Source: CAD feature listing. Evaluate the final solid. Frame: model axes, mm. A direction names the side the tool comes from. Round coordinates to 2 decimals unless told otherwise and drop trailing zeros. Order: outer loops, then holes, each group sorted by start corner. A loop starts at its lowest first (then second) coordinate and runs counter-clockwise, first axis right, second up. Notation, with made-up numbers: M 73,36 L 102,36 A22 ccw 102,42 Z; hole C -31,11.5 d9. An arc over 180 degrees is marked long. Answer in a Markdown table with one row per item. Add a question column.
```python
from build123d import *

# Parameters (mm, degrees)
SKETCH1_R          = 0.75
BASE_FLANGE1_DEPTH = 1


# Sheet-metal steps are written as plain solids
with BuildPart() as part:
    # Sketch1 → Base-Flange1 (new body)
    with BuildSketch(Plane.XY):
        with BuildLine():
            Line((-3.140050919, -11.322657825), (-2.47867317, -8.937806709))
            ThreePointArc((-2.47867317, -8.937806709), (-2.938495148, -7.231063808), (-4.684207754, -6.95376419))
            ThreePointArc((-4.684207754, -6.95376419), (-7.062092174, -7.07208067), (-8.90450501, -5.564152274))
            ThreePointArc((-8.90450501, -5.564152274), (0, 9.743819977), (8.90450501, -5.564152274))
            ThreePointArc((8.90450501, -5.564152274), (7.062092174, -7.07208067), (4.684207754, -6.95376419))
            ThreePointArc((4.684207754, -6.95376419), (2.938495148, -7.231063808), (2.47867317, -8.937806709))
            Line((2.47867317, -8.937806709), (3.140050919, -11.322657825))
            ThreePointArc((3.140050919, -11.322657825), (0, 11.75), (-3.140050919, -11.322657825))
        make_face()
        with Locations((-4.025278755, -8.439172409)):
            Circle(SKETCH1_R, mode=Mode.SUBTRACT)
        with Locations(Location((4.025278755, -8.439172409, 0), (0, 0, 180))):
            Circle(SKETCH1_R, mode=Mode.SUBTRACT)
    extrude(amount=-BASE_FLANGE1_DEPTH)


solid = part.part
```
(1) Cut plane A-A (y = 3.5). Return loops of the section in (x, z).
(2) Cut plane D-D (y = -8). Return loops of the section in (x, z), and give its area (3 significant figures).
(3) Access query for faces 1 (the face through (7.094, -7.061, -0.493)), 2 (the face through (-4, -7, -1)), 3 (the face through (2.8, -10.1, -0.5)). Directions: +Z, -Z, +X, -X, +Y, -Y. A direction counts if a zero-diameter tool reaches every point of the face in a straight line with its end or side. Return the directions, or none.
(4) Line query: line 1 (X direction, y = -9, z = -0.9); line 2 (X direction, y = -8.75, z = -0.75); line 3 (Y direction, x = -9, z = -0.4). Output: solid intervals per line, ascending. Write a range as from..to.
(5) Cut plane B-B (x = 9.75). Return loops of the section in (y, z).
(6) Draft query along X for faces 4 (the face through (0.47, 11.74, -0.49)), 5 (the face through (-2.92, -7.25, -0.49)), 6 (the face through (-4, -7, 0)). Return one class per face: +X half, -X half, draft (parallel to the pull), parting line (faces both ways), or undercut.
(7) Cut plane C-C (x = 4.25). Return loops of the section in (y, z).
Answer list:
| question | item | result |
|---|---|---|
| 1 | outline | M -11.22,-1 L -9.43,-1 L -9.43,0 L -11.22,0 Z; M 9.43,-1 L 11.22,-1 L 11.22,0 L 9.43,0 Z |
| 2 | outline | M -8.61,-1 L -4.63,-1 L -4.63,0 L -8.61,0 Z; M -3.42,-1 L -2.46,-1 L -2.46,0 L -3.42,0 Z; M 2.46,-1 L 3.42,-1 L 3.42,0 L 2.46,0 Z; M 4.63,-1 L 8.61,-1 L 8.61,0 L 4.63,0 Z |
| 2 | area | 9.86 mm² |
| 3 | face 1 | +Z, -Z |
| 3 | face 2 | -Z, +X, -X, +Y, -Y |
| 3 | face 3 | +Z, -Z, -Y |
| 4 | line 1 | -7.55..-4.52, -3.53..-2.5, 2.5..3.53, 4.52..7.55 |
| 4 | line 2 | -7.84..-4.71, -3.34..-2.43, 2.43..3.34, 4.71..7.84 |
| 4 | line 3 | -7.55..-5.39, 4.39..7.55 |
| 5 | outline | M -6.56,-1 L -3.64,-1 L -3.64,0 L -6.56,0 Z; M 2.64,-1 L 6.56,-1 L 6.56,0 L 2.64,0 Z |
| 6 | face 4 | parting line |
| 6 | face 5 | undercut |
| 6 | face 6 | draft |
| 7 | outline | M -10.95,-1 L -9.15,-1 L -9.15,0 L -10.95,0 Z; M -7.72,-1 L -6.83,-1 L -6.83,0 L -7.72,0 Z; M 8.82,-1 L 10.95,-1 L 10.95,0 L 8.82,0 Z |
